Source: CAD feature listing. Evaluate the final solid. Frame: model axes, mm. Round coordinates to 2 decimals unless told otherwise and drop trailing zeros. Write each loop counter-clockwise with the first axis right and the second up, starting at its lowest first coordinate (ties: lowest second). Pieces come first, ordered by that corner, then holes. Notation, with made-up numbers: M 57,40 L 112,40 A15 ccw 112,65 Z; hole C 85.25,75 d3. An arc over 180 degrees is marked long. Answer in a Markdown table with one row per item. Add a question column.
Item 1: Contact query for a flat-ended pin moving along its axis: pin 1 (3 mm diameter, centred on x = 62, y = 35.39, fed in from -Z). Output: stop coordinate, or through.
Item 2: Cut plane A-A on y = -35.5. Return loops of the section in (x, z), and give its area (4 significant figures).
Item 3: Material intervals for probe 1 along Y at (x, z) = (-60.1, 25.95); probe 2 along Y at (x, z) = (-61, 24.9), sorted ascending.
Item 4: Cut plane B-B on x = -60.1. Return loops of the section in (y, z), and give its area (3 significant figures).
Solid Edge part; units mm, degrees
sketch "Sketch1" plane through (0, 0, 22) normal (0, 0, 1) x (1, 0, 0)
  circle A0 centre (62, 35.3919) radius 1.7
  circle A1 centre (62, -35.5) radius 1.7
  circle A2 centre (-60.1, -35.5) radius 1.7
  line L0 (-68.1, -70) -> (70, -70)
  line L1 (70, -70) -> (70, 70)
  line L2 (70, 70) -> (-68.1, 70)
  line L3 (-68.1, 70) -> (-68.1, -70)
  circle A3 centre (-60.1, 35.3919) radius 1.7
  dimension "D1" = 62
  dimension "D2" = 68.1
extrude "ExtrudedProtrusion_1" add sketch "Sketch1" along normal blind 5
properties material "Steel"
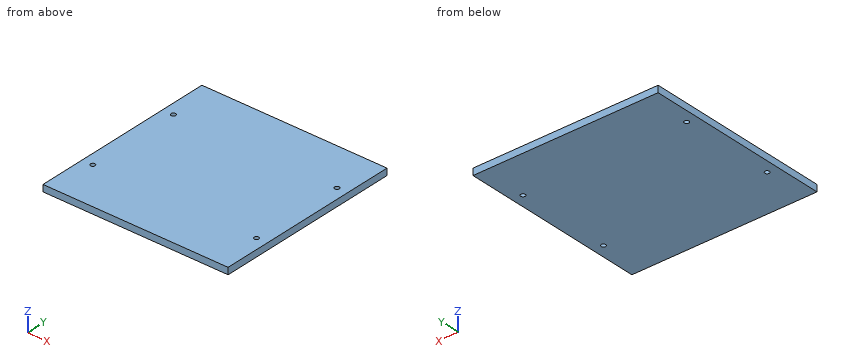
Results below:
| question | item | result |
|---|---|---|
| 1 | pin 1 | through |
| 2 | outline | M -68.1,22 L -61.8,22 L -61.8,27 L -68.1,27 Z; M -58.4,22 L 60.3,22 L 60.3,27 L -58.4,27 Z; M 63.7,22 L 70,22 L 70,27 L 63.7,27 Z |
| 2 | area | 656.5 mm2 |
| 3 | probe 1 | -70 to -37.2, -33.8 to 33.69, 37.09 to 70 |
| 3 | probe 2 | -70 to -36.94, -34.06 to 33.95, 36.83 to 70 |
| 4 | outline | M -70,22 L -37.2,22 L -37.2,27 L -70,27 Z; M -33.8,22 L 33.69,22 L 33.69,27 L -33.8,27 Z; M 37.09,22 L 70,22 L 70,27 L 37.09,27 Z |
| 4 | area | 666 mm2 |
